```python
from build123d import *

# Parameters (mm, degrees)
F0_W     = 101.6
F0_H     = 12.7
F1_DEPTH = 6.4
F2_DEPTH = 31.7
F3_DEPTH = 6.4
F4_R     = 5


with BuildPart() as f1:
    # F0 (on Top) → F1 (new body)
    with BuildSketch(Plane.XY):
        Polygon((-25.4, -88.9), (50.8, -88.9), (50.8, -10.749764), (50.8, 0), (-25.4, 0), align=None)
        with BuildLine():
            ThreePointArc((33.332847, -10.749764), (38.332847, -5.749764), (43.332847, -10.749764))
            Line((43.332847, -10.749764), (43.332847, -61.549764))
            ThreePointArc((43.332847, -61.549764), (38.332847, -66.549764), (33.332847, -61.549764))
            Line((33.332847, -61.549764), (33.332847, -10.749764))
        make_face(mode=Mode.SUBTRACT)
        Polygon((-50.8, -88.9), (-25.4, -88.9), (-25.4, 0), (50.8, 0), (50.8, 76.2), (-50.8, 76.2), (-50.8, -10.067825), align=None)
        with BuildLine():
            Line((-43.099635, -60.867813), (-43.099635, -10.067825))
            ThreePointArc((-43.099635, -10.067825), (-38.08229, -5.067855), (-33.099755, -10.102513))
            Line((-33.099755, -10.102513), (-33.099635, -60.867813))
            ThreePointArc((-33.099635, -60.867813), (-38.099635, -65.867813), (-43.099635, -60.867813))
        make_face(mode=Mode.SUBTRACT)
        with BuildLine():
            Line((-33.099635, 66.132175), (-33.099635, 15.332175))
            ThreePointArc((-33.099635, 15.332175), (-38.099635, 10.332175), (-43.099635, 15.332175))
            Line((-43.099635, 15.332175), (-43.099635, 66.132175))
            ThreePointArc((-43.099635, 66.132175), (-38.099635, 71.132175), (-33.099635, 66.132175))
        make_face(mode=Mode.SUBTRACT)
        with BuildLine():
            Line((43.100365, 66.132175), (43.100365, 15.332175))
            ThreePointArc((43.100365, 15.332175), (38.100365, 10.332175), (33.100365, 15.332175))
            Line((33.100365, 15.332175), (33.100365, 66.132175))
            ThreePointArc((33.100365, 66.132175), (38.100365, 71.132175), (43.100365, 66.132175))
        make_face(mode=Mode.SUBTRACT)
        with Locations((0, 82.55)):
            Rectangle(F0_W, F0_H)
    extrude(amount=-F1_DEPTH)

    # F0 (on Top) → F2 (join)
    with BuildSketch(Plane.XY):
        with Locations((0, 82.55)):
            Rectangle(F0_W, F0_H)
    extrude(amount=F2_DEPTH)

    # F0 (on Top) → F3 (cut)
    with BuildSketch(Plane.XY):
        Polygon((-25.4, -88.9), (50.8, -88.9), (50.8, -10.749764), (50.8, 0), (-25.4, 0), align=None)
        with BuildLine():
            ThreePointArc((33.332847, -10.749764), (38.332847, -5.749764), (43.332847, -10.749764))
            Line((43.332847, -10.749764), (43.332847, -61.549764))
            ThreePointArc((43.332847, -61.549764), (38.332847, -66.549764), (33.332847, -61.549764))
            Line((33.332847, -61.549764), (33.332847, -10.749764))
        make_face(mode=Mode.SUBTRACT)
    extrude(amount=-F3_DEPTH, mode=Mode.SUBTRACT)

    # F4
    f4_edges = [f1.edges().sort_by_distance(p)[0] for p in [
        (0, 76.2, 0),
        (50.8, 88.9, 12.65),
        (-50.8, 88.9, 12.65),
        (50.8, 0, -3.2),
        (-25.4, 0, -3.2),
        (-25.4, -88.9, -3.2),
        (-50.8, -88.9, -3.2),
    ]]
    fillet(f4_edges, radius=F4_R)


solid = f1.part
```
Check sheet for the modelled part. Datum: model origin and axes. Units: mm. A direction names the side the tool comes from. Round coordinates to 2 decimals unless told otherwise and drop trailing zeros. Order: outer loops, then holes, each group sorted by start corner. A loop starts at its lowest first (then second) coordinate and runs counter-clockwise, first axis right, second up. Notation, with made-up numbers: (11, 3) - (56, 3) arc R23 cw to (56, 18) - close; hole circle Ø4 at (87.5, -30.5). An arc over 180 degrees is marked (long way). Write item = value, one per line.
Q1. Section check C-C (y = -19). Record the boundary of the cut face in (x, z), and give its area (3 significant figures).
Computed:
outline = (-50.8, -6.4) - (-43.1, -6.4) - (-43.1, 0) - (-50.8, 0) - close; (-33.1, -6.4) - (-25.4, -6.4) - (-25.4, 0) - (-33.1, 0) - close
area = 98.6 mm^2
Q2. Section check B-B (x = -35). Record the boundary of the cut face in (y, z), and give its area (3 significant figures).
Computed:
outline = (-88.9, -6.4) - (-64.79, -6.4) - (-64.79, 0) - (-88.9, 0) - close; (-6.14, -6.4) - (11.41, -6.4) - (11.41, 0) - (-6.14, 0) - close; (70.06, -6.4) - (88.9, -6.4) - (88.9, 31.7) - (76.2, 31.7) - (76.2, 5) arc R5 cw to (71.2, 0) - (70.06, 0) - close
area = 795 mm^2
Q3. Go/stop test with flat-tipped pins: pin 1 (5 mm diameter, centred on y = -35.5, z = -2, fed in from +X); pin 2 (8 mm diameter, centred on x = 24, z = 20.5, fed in from -Y); pin 3 (1.9 mm diameter, centred on x = 1.5, z = -4.5, fed in from -Y). Record where each tip stops, or that it passes through.
Computed:
pin_1 = -25.4
pin_2 = 76.2
pin_3 = 0
Q4. Thickness scan on line 1 along Y through (x, z) = (-26.5, 7); line 2 along Z through (x, y) = (-42, -80); line 3 along Y through (x, z) = (-21, -3.5). Record the ranges inside material, lowest first.
Computed:
line_1 = 76.2 to 88.9
line_2 = -6.4 to 0
line_3 = -0.04 to 88.9
Q5. Section check D-D (x = -11.5). Record the boundary of the cut face in (y, z).
Computed:
outline = (0, -6.4) - (88.9, -6.4) - (88.9, 31.7) - (76.2, 31.7) - (76.2, 5) arc R5 cw to (71.2, 0) - (0, 0) - close
Q6. Draft check along X on faces 1 (the face through (-26.9, -87.47, -3.24)), 2 (the face through (-49.37, 87.4, 12.38)), 3 (the face through (-33.1, 41, -3)), 4 (the face through (-1, 83, 31.7)). Enter one of: pulls with the +X half, pulls with the -X half, needs draft (parallel to the pull), parting line crosses it, or undercut.
Computed:
face_1 = pulls with the +X half
face_2 = pulls with the -X half
face_3 = undercut
face_4 = needs draft
Q7. Section check A-A (z = -3). Record the boundary of the cut face in (x, y).
Computed:
outline = (-50.8, -83.9) arc R5 ccw to (-45.8, -88.9) - (-30.4, -88.9) arc R5 ccw to (-25.4, -83.9) - (-25.4, -5) arc R5 cw to (-20.4, 0) - (45.8, 0) arc R5 ccw to (50.8, 5) - (50.8, 83.9) arc R5 ccw to (45.8, 88.9) - (-45.8, 88.9) arc R5 ccw to (-50.8, 83.9) - close; hole (-43.1, -60.87) arc R5 ccw to (-33.1, -60.87) - (-33.1, -10.1) arc R5 ccw (long way) to (-43.1, -10.07) - close; hole (-43.1, 15.33) arc R5 ccw to (-33.1, 15.33) - (-33.1, 66.13) arc R5 ccw to (-43.1, 66.13) - close; hole (33.1, 15.33) arc R5 ccw to (43.1, 15.33) - (43.1, 66.13) arc R5 ccw to (33.1, 66.13) - close
Q8. Tool access check on faces 5 (the face through (-25.4, -44, -3)), 6 (the face through (50.8, 56, -3)), 7 (the face through (-12, 28, 0)), 8 (the face through (-38.19, -5.07, -3.16)), 9 (the face through (-1, 21, -6.4)). Record the directions out of +Z, -Z, +X, -X, +Y, -Y that give a thin tool (end or side, any length) a straight path to the whole face; none if there is none.
Computed:
face_5 = +Z, -Z, +X, -Y
face_6 = +Z, -Z, +X, +Y, -Y
face_7 = +Z, +X, -X, -Y
face_8 = +Z, -Z
face_9 = -Z, +X, -X, +Y, -Y
